The model under review builds one solid part; all positions refer to its coordinate system, in mm. Face numbers are marked on the shaded views. A direction names the side the tool comes from. Coordinates: 2 decimals unless noted, no trailing zeros. Write each loop counter-clockwise with the first axis right and the second up, starting at its lowest first coordinate (ties: lowest second). Pieces come first, ordered by that corner, then holes. Notation, with made-up numbers: (13, 43.25) - (58, 43.25) arc R27 cw to (58, 73.25) - close; hole circle Ø8 at (32.25, 21). An arc over 180 degrees is marked (long way). Answer as CSV lines item,"result". Start each with the question number.
Autodesk Inventor part; units mm, degrees
ref_plane "YZ Plane" through (0, 0, 0) normal (1, 0, 0) x (0, 1, 0)
ref_plane "XZ Plane" through (0, 0, 0) normal (0, 1, 0) x (-1, 0, 0)
ref_plane "XY Plane" through (0, 0, 0) normal (0, 0, 1) x (1, 0, 0)
sketch "Sketch1" plane through (0, 0, 0) normal (0, 1, 0) x (-1, 0, 0)
  circle A0 centre (0, 0) radius 254
  dimension "d0" = 508
extrude "Extrusion1" add sketch "Sketch1" along normal blind 25.4
sketch "Sketch2" plane through (0, 25.4, 0) normal (0, 1, 0) x (1, 0, 0)
  circle A0 centre (0, 0) radius 139.7
  dimension "d3" = 279.4
extrude "Extrusion2" add sketch "Sketch2" along normal blind 50.8
sketch "Sketch3" plane through (0, 0, 0) normal (0, 1, 0) x (-1, 0, 0)
  circle A0 centre (0, 0) radius 133.35
  dimension "d6" = 266.7
extrude "Extrusion3" cut sketch "Sketch3" along normal up to next
sketch "Sketch4" plane through (0, 0, 0) normal (0, 0, 1) x (1, 0, 0)
  circle A0 centre (0, 50.8) radius 6.35
  line L0 (254, 25.4) -> (-254, 25.4)
  point P0 (0, 0)
  dimension "d9" = 12.7
  dimension "d10" = 25.4
extrude "Extrusion4" cut sketch "Sketch4" along normal mid plane 228.6
sketch "Sketch5" plane through (0, 0, 0) normal (0, 0, 1) x (1, 0, 0)
  circle A0 centre (0, 47.8947) radius 6.35
  point P0 (0, 0)
  dimension "d13" = 12.7
extrude "Extrusion5" cut sketch "Sketch5" along normal mid plane 381
properties part number "Top2"
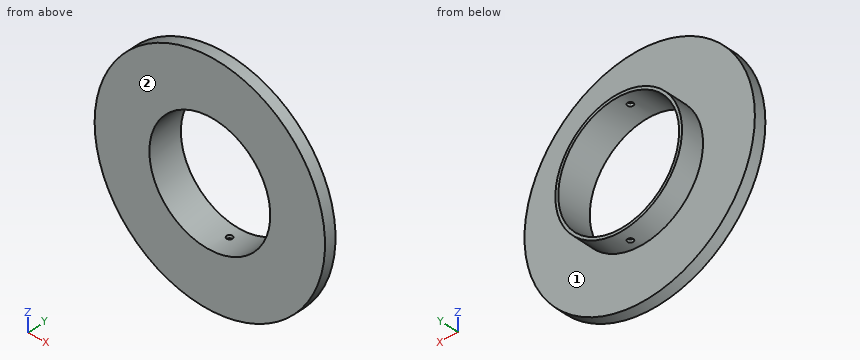
(1) Add section C-C on x = 87.5. Give the boundary of the cut face in (y, z).
(2) For pin 1 (5 mm diameter, centred on x = 159.5, z = -193.5, fed in from +Y); pin 2 (1.5 mm diameter, centred on x = 97.5, y = 11, fed in from +Z); pin 3 (8 mm diameter, centred on x = 143.5, z = -118.5, fed in from -Y); pin 4 (6 mm diameter, centred on y = 67, z = -43.5, fed in from -X), all flat-tipped, find the tip position at first contact; note any pin that passes through.
(3) For the marked faces 1 and 2, list the 3-axis set-ups (+Z, -Z, +X, -X, +Y, -Y) from which the entire face can be reached by the end or side of a thin tool; tool diameter is ignored.
(4) Add section B-B on x = 0. Give the boundary of the cut face in (y, z).
(5) Wall thickness on line 1 (X direction, y = 35.5, z = 0); line 2 (Y direction, x = 0, z = -134); line 3 (Z direction, x = 5.5, y = 65.5): over which ranges is each line inside the solid? List them lowest first.
(6) Add section D-D on y = 67.5. Give the boundary of the cut face in (x, z).
(7) Add section A-A on z = 0. Give the boundary of the cut face in (x, y), then the cut area to 3 significant figures.
Reported:
1,outline,"(0, -238.45) - (25.4, -238.45) - (25.4, -108.9) - (76.2, -108.9) - (76.2, -100.63) - (0, -100.63) - close; (0, 100.63) - (76.2, 100.63) - (76.2, 108.9) - (25.4, 108.9) - (25.4, 238.45) - (0, 238.45) - close"
2,pin 1,"y = 25.4"
2,pin 2,"z = 234.85"
2,pin 3,"y = 0"
2,pin 4,"x = -133.7"
3,face 1,"+Y"
3,face 2,"+Z, -Z, +X, -X, -Y"
4,outline,"(0, -254) - (25.4, -254) - (25.4, -139.7) - (41.54, -139.7) - (41.54, -133.35) - (0, -133.35) - close; (0, 133.35) - (41.54, 133.35) - (41.54, 139.7) - (25.4, 139.7) - (25.4, 254) - (0, 254) - close; (54.24, -139.7) - (76.2, -139.7) - (76.2, -133.35) - (54.24, -133.35) - close; (54.24, 133.35) - (76.2, 133.35) - (76.2, 139.7) - (54.24, 139.7) - close"
5,line 1,"-139.7 to -133.35, 133.35 to 139.7"
5,line 2,"0 to 41.54, 54.24 to 76.2"
5,line 3,"-139.59 to -133.24, 133.24 to 139.59"
6,outline,"circle Ø279.4 at (0, 0); hole circle Ø266.7 at (0, 0)"
7,outline,"(-254, 0) - (-133.35, 0) - (-133.35, 76.2) - (-139.7, 76.2) - (-139.7, 25.4) - (-254, 25.4) - close; (133.35, 0) - (254, 0) - (254, 25.4) - (139.7, 25.4) - (139.7, 76.2) - (133.35, 76.2) - close"
7,area,"6,770 mm²"
